```python
from build123d import *

# Parameters (mm, degrees)
CUT_EXTRUDE2_DEPTH = 21.5
SKETCH4_R          = 4
CUT_EXTRUDE3_DEPTH = 6.7
SKETCH5_R          = 4
CUT_EXTRUDE4_DEPTH = 36.7
CIRPATTERN1_COUNT  = 4
CUT_EXTRUDE5_DEPTH = 0.5


with BuildPart() as part:
    # Sketch1 → Revolve1 (revolve)
    with BuildSketch(Plane.XY):
        Polygon((16.25, -33.807578124), (29.5, -33.807578124), (29.5, -31.007578124), (43.5, -31.007578124), (43.5, -21.007578124), (29.5, -21.007578124), (29.5, -16.800812474), (27.5, -16.800812474), (27.5, -14.000812474), (29.5, -14.000812474), (29.5, -10.507578124), (22.5, -10.507578124), (22.5, -25.507578124), (16.25, -25.507578124), align=None)
    revolve(axis=Axis((0, 0, 0), (0, -1, 0)))

    # Sketch2 → Cut-Extrude2 (cut, through all)
    with BuildSketch(Plane.XZ.offset(31.007578124)):
        with BuildLine():
            ThreePointArc((-36.006849315, 5.97969919), (-34.394339083, 12.217996522), (-31.710007458, 18.075547766))
            ThreePointArc((-31.710007458, 18.075547766), (-31.185597591, 20.120976666), (-31.775738857, 22.148418004))
            ThreePointArc((-31.775738857, 22.148418004), (-32.761116978, 26.630126752), (-30.759144987, 30.759144976))
            ThreePointArc((-30.759144987, 30.759144976), (-43.5, -2.1e-08), (-30.759144958, -30.759145005))
            ThreePointArc((-30.759144958, -30.759145005), (-32.761116976, -26.630126773), (-31.775738857, -22.148418004))
            ThreePointArc((-31.775738857, -22.148418004), (-31.185597591, -20.120976666), (-31.710007458, -18.075547766))
            ThreePointArc((-31.710007458, -18.075547766), (-34.394339083, -12.217996522), (-36.006849315, -5.97969919))
            ThreePointArc((-36.006849315, -5.97969919), (-42.5, 0), (-36.006849315, 5.97969919))
        make_face()
        with BuildLine():
            ThreePointArc((-22.148418004, 31.775738857), (-20.120976666, 31.185597591), (-18.075547766, 31.710007458))
            ThreePointArc((-18.075547766, 31.710007458), (-12.217996522, 34.394339083), (-5.97969919, 36.006849315))
            ThreePointArc((-5.97969919, 36.006849315), (0, 42.5), (5.97969919, 36.006849315))
            ThreePointArc((5.97969919, 36.006849315), (12.217996522, 34.394339083), (18.075547766, 31.710007458))
            ThreePointArc((18.075547766, 31.710007458), (20.120976666, 31.185597591), (22.148418004, 31.775738857))
            ThreePointArc((22.148418004, 31.775738857), (26.630126737, 32.76111698), (30.759144954, 30.759145009))
            ThreePointArc((30.759144954, 30.759145009), (-2.4e-08, 43.5), (-30.759144987, 30.759144976))
            ThreePointArc((-30.759144987, 30.759144976), (-26.63012676, 32.761116977), (-22.148418004, 31.775738857))
        make_face()
        with BuildLine():
            ThreePointArc((30.759144986, -30.759144977), (43.5, 2.3e-08), (30.759144954, 30.759145009))
            ThreePointArc((30.759144954, 30.759145009), (32.761116975, 26.630126776), (31.775738857, 22.148418004))
            ThreePointArc((31.775738857, 22.148418004), (31.185597591, 20.120976666), (31.710007458, 18.075547766))
            ThreePointArc((31.710007458, 18.075547766), (34.394339083, 12.217996522), (36.006849315, 5.97969919))
            ThreePointArc((36.006849315, 5.97969919), (42.5, 0), (36.006849315, -5.97969919))
            ThreePointArc((36.006849315, -5.97969919), (34.394339083, -12.217996522), (31.710007458, -18.075547766))
            ThreePointArc((31.710007458, -18.075547766), (31.185597591, -20.120976666), (31.775738857, -22.148418004))
            ThreePointArc((31.775738857, -22.148418004), (32.761116978, -26.630126753), (30.759144986, -30.759144977))
        make_face()
        with BuildLine():
            ThreePointArc((-22.148418004, -31.775738857), (-26.630126739, -32.76111698), (-30.759144958, -30.759145005))
            ThreePointArc((-30.759144958, -30.759145005), (2e-08, -43.5), (30.759144986, -30.759144977))
            ThreePointArc((30.759144986, -30.759144977), (26.630126759, -32.761116977), (22.148418004, -31.775738857))
            ThreePointArc((22.148418004, -31.775738857), (20.120976666, -31.185597591), (18.075547766, -31.710007458))
            ThreePointArc((18.075547766, -31.710007458), (12.217996522, -34.394339083), (5.97969919, -36.006849315))
            ThreePointArc((5.97969919, -36.006849315), (0, -42.5), (-5.97969919, -36.006849315))
            ThreePointArc((-5.97969919, -36.006849315), (-12.217996522, -34.394339083), (-18.075547766, -31.710007458))
            ThreePointArc((-18.075547766, -31.710007458), (-20.120976666, -31.185597591), (-22.148418004, -31.775738857))
        make_face()
    extrude(amount=-CUT_EXTRUDE2_DEPTH, mode=Mode.SUBTRACT)

    # Sketch4 → Cut-Extrude3 (cut)
    with BuildSketch(Plane.XZ.offset(31.007578124)):
        with BuildLine():
            ThreePointArc((20.120976666, 31.185597591), (18.564665358, 25.884871335), (20.859650045, 20.859650045))
            ThreePointArc((20.859650045, 20.859650045), (25.884871335, 18.564665358), (31.185597591, 20.120976666))
            ThreePointArc((31.185597591, 20.120976666), (31.344468449, 21.174341938), (31.775738857, 22.148418004))
            ThreePointArc((31.775738857, 22.148418004), (30.759144982, 30.759144982), (22.148418004, 31.775738857))
            ThreePointArc((22.148418004, 31.775738857), (21.174341938, 31.344468449), (20.120976666, 31.185597591))
        make_face()
        with Locations((25.809397513, 25.809397513)):
            Circle(SKETCH4_R, mode=Mode.SUBTRACT)
    cut_extrude3 = extrude(amount=-CUT_EXTRUDE3_DEPTH, mode=Mode.SUBTRACT)

    # Sketch5 → Cut-Extrude4 (cut)
    with BuildSketch(Plane.XZ.offset(31.007578124)):
        with Locations((25.809397513, 25.809397513)):
            Circle(SKETCH5_R)
    cut_extrude4 = extrude(amount=-CUT_EXTRUDE4_DEPTH, mode=Mode.SUBTRACT)

    # CirPattern1: Cut-Extrude3, Cut-Extrude4 ×4 about axis
    cirpattern1_axis = Axis((0, 0, 0), (0, 1, 0))
    for i in range(1, CIRPATTERN1_COUNT):
        add(cut_extrude3.rotate(cirpattern1_axis, i * 360 / CIRPATTERN1_COUNT), mode=Mode.SUBTRACT)
        add(cut_extrude4.rotate(cirpattern1_axis, i * 360 / CIRPATTERN1_COUNT), mode=Mode.SUBTRACT)

    # Sketch6 → Cut-Extrude5 (cut)
    with BuildSketch(Plane(origin=(0, -10.507578124, 0), x_dir=(1, 0, 0), z_dir=(0, 1, 0))):
        with BuildLine():
            Line((21.162631221, 18.334204096), (19.035223749, 16.206796624))
            ThreePointArc((19.035223749, 16.206796624), (22.692759246, 10.489932212), (24.677925359, 4))
            Line((24.677925359, 4), (27.712812921, 4))
            ThreePointArc((27.712812921, 4), (25.467029897, 11.637456261), (21.162631221, 18.334204096))
        make_face()
        with BuildLine():
            ThreePointArc((4, 24.677925359), (10.489932212, 22.692759246), (16.206796624, 19.035223749))
            Line((16.206796624, 19.035223749), (18.334204096, 21.162631221))
            ThreePointArc((18.334204096, 21.162631221), (11.637456261, 25.467029897), (4, 27.712812921))
            Line((4, 27.712812921), (4, 24.677925359))
        make_face()
        with BuildLine():
            Line((19.035223749, -16.206796624), (21.162631221, -18.334204096))
            ThreePointArc((21.162631221, -18.334204096), (25.467029897, -11.637456261), (27.712812921, -4))
            Line((27.712812921, -4), (24.677925359, -4))
            ThreePointArc((24.677925359, -4), (22.692759246, -10.489932212), (19.035223749, -16.206796624))
        make_face()
        with BuildLine():
            Line((18.334204096, -21.162631221), (16.206796624, -19.035223749))
            ThreePointArc((16.206796624, -19.035223749), (10.489932212, -22.692759246), (4, -24.677925359))
            Line((4, -24.677925359), (4, -27.712812921))
            ThreePointArc((4, -27.712812921), (11.637456261, -25.467029897), (18.334204096, -21.162631221))
        make_face()
        with BuildLine():
            Line((-4, 24.677925359), (-4, 27.712812921))
            ThreePointArc((-4, 27.712812921), (-19.798989873, 19.798989873), (-27.712812921, 4))
            Line((-27.712812921, 4), (-24.677925359, 4))
            ThreePointArc((-24.677925359, 4), (-17.67766953, 17.67766953), (-4, 24.677925359))
        make_face()
        with BuildLine():
            Line((-24.677925359, -4), (-27.712812921, -4))
            ThreePointArc((-27.712812921, -4), (-25.467029897, -11.637456261), (-21.162631221, -18.334204096))
            Line((-21.162631221, -18.334204096), (-19.035223749, -16.206796624))
            ThreePointArc((-19.035223749, -16.206796624), (-22.692759246, -10.489932212), (-24.677925359, -4))
        make_face()
        with BuildLine():
            Line((-16.206796624, -19.035223749), (-18.334204096, -21.162631221))
            ThreePointArc((-18.334204096, -21.162631221), (-11.637456261, -25.467029897), (-4, -27.712812921))
            Line((-4, -27.712812921), (-4, -24.677925359))
            ThreePointArc((-4, -24.677925359), (-10.489932212, -22.692759246), (-16.206796624, -19.035223749))
        make_face()
    extrude(amount=-CUT_EXTRUDE5_DEPTH, mode=Mode.SUBTRACT)


solid = part.part
```
Part model, mm, in its own coordinate system. A direction names the side the tool comes from. Give positions to 0.01 mm unless a question says otherwise; leave off trailing zeros. Order: outer loops, then holes, each group sorted by start corner. A loop starts at its lowest first (then second) coordinate and runs counter-clockwise, first axis right, second up. Notation, with made-up numbers: (2.25, 12) - (58.25, 12) arc R19 ccw to (58.25, 46) - close; hole circle Ø9 at (-12, -8). An arc over 180 degrees is marked (long way). Use one line per item in the form item = value.
Item 1: Which spindle directions (+Z, -Z, +X, -X, +Y, -Y) get a long thin tool onto all of the face, cutting with end or side? Do faces 4 (the face through (31.2, -25, 19.7)), 5 (the face through (11, -11.008, -23)). Say none if no direction does.
Solution:
face_4 = +X, +Y, -Y
face_5 = +Y
Item 2: Slice it at A-A on z = 0. Give the cut face in (x, y), and give its area (3 significant figures).
Solution:
outline = (-42.5, -31.01) - (-29.5, -31.01) - (-29.5, -33.81) - (-16.25, -33.81) - (-16.25, -25.51) - (-22.5, -25.51) - (-22.5, -10.51) - (-29.5, -10.51) - (-29.5, -14) - (-27.5, -14) - (-27.5, -16.8) - (-29.5, -16.8) - (-29.5, -21.01) - (-42.5, -21.01) - close; (16.25, -33.81) - (29.5, -33.81) - (29.5, -31.01) - (42.5, -31.01) - (42.5, -21.01) - (29.5, -21.01) - (29.5, -16.8) - (27.5, -16.8) - (27.5, -14) - (29.5, -14) - (29.5, -10.51) - (22.5, -10.51) - (22.5, -25.51) - (16.25, -25.51) - close
area = 679 mm2
Item 3: Slice it at B-B on x = 0. Give the cut face in (y, z), and give its area (3 significant figures).
Solution:
outline = (-33.81, -29.5) - (-31.01, -29.5) - (-31.01, -42.5) - (-21.01, -42.5) - (-21.01, -29.5) - (-16.8, -29.5) - (-16.8, -27.5) - (-14, -27.5) - (-14, -29.5) - (-10.51, -29.5) - (-10.51, -22.5) - (-25.51, -22.5) - (-25.51, -16.25) - (-33.81, -16.25) - close; (-33.81, 16.25) - (-25.51, 16.25) - (-25.51, 22.5) - (-10.51, 22.5) - (-10.51, 29.5) - (-14, 29.5) - (-14, 27.5) - (-16.8, 27.5) - (-16.8, 29.5) - (-21.01, 29.5) - (-21.01, 42.5) - (-31.01, 42.5) - (-31.01, 29.5) - (-33.81, 29.5) - close
area = 679 mm2
Item 4: Slice it at D-D on z = -37. Give the cut face in (x, y).
Solution:
outline = (-5.98, -31.01) - (5.98, -31.01) - (5.98, -21.01) - (-5.98, -21.01) - close
Item 5: Slice it at C-C on y = -32. Give the cut face in (x, z).
Solution:
outline = circle Ø59 at (0, 0); hole circle Ø32.5 at (0, 0)
Item 6: Probe probe 1 along X at (y, z) = (-23, -31.5); probe 2 along Y at (x, z) = (29.5, -19); probe 3 along X at (y, z) = (-30.25, 13.5). List the from-to ranges inside material, lowest first. Write a range as from..to.
Solution:
probe_1 = -29.89..-21.61, -18.5..18.5, 21.61..29.89
probe_2 = -31.01..-21.01
probe_3 = -33.91..-9.05, 9.05..33.91
Item 7: Two-plate mould, pull along Z, no slides. Class faces 1 (the face through (32, -31.008, 0)), 2 (the face through (-42.5, -26.1, -0.1)), 3 (the face through (-31.21, -24.97, 19.62)): released by +Z, released by -Z, zero draft, split by the parting line, or undercut.
Solution:
face_1 = zero draft
face_2 = split by the parting line
face_3 = undercut
Item 8: Pin check, flat tips, straight feed: pin 1 Ø15.5 at (x, z) = (-29, 28) entering from -Y; pin 2 Ø4 at (x, y) = (-31, -20) entering from +Z; pin 3 Ø4 at (x, z) = (-11.5, 28.5) entering from -Y; pin 4 Ø12 at (x, y) = (-25, -16) entering from -Z. Stop position of each tip, or through.
Solution:
pin_1 = -24.31
pin_2 = 31.89
pin_3 = -33.81
pin_4 = -32.81
